```python
from build123d import *

# Parameters (mm, degrees)
F0_W        = 34.925
F0_H        = 25.4
F1_DEPTH    = 3.1496
F2_SIZE     = 3.14959
F3_W        = 29.1948509403
F3_H        = 13.3209023625
F4_DEPTH    = 25.4
F5_T        = 2.54
F5_T3_DEPTH = 34.2748509403
F5_T5_DEPTH = 18.4009023625


# Not quite as in the source:
# - a fillet or chamfer is up to 0.001 mm smaller than in the source, because OpenCascade refuses the exact size
# - a shell that OpenCascade refuses in one call is made with other operations: the cavity is built on its own and cut out


with BuildPart() as f1:
    # F0 (on Top) → F1 (new body)
    with BuildSketch(Plane.XY):
        with Locations((9.7498925388, -19.8326882303)):
            Rectangle(F0_W, F0_H)
    extrude(amount=F1_DEPTH)

    # F2 (size 3.1496 in the source; OpenCascade refuses exactly that, so slightly less here)
    f2_edges = [f1.edges().sort_by_distance(p)[0] for p in [
        (9.749893, -32.532688, 3.1496),
        (9.749893, -7.132688, 3.1496),
    ]]
    chamfer(f2_edges, length=F2_SIZE)

    # F3 (on face) → F4 (join)
    with BuildSketch(Plane.XY.offset(3.1496)):
        with Locations((8.8992563542, -19.3738183007)):
            Rectangle(F3_W, F3_H)
    extrude(amount=F4_DEPTH)

    # F5: shell of thickness 2.54, made by hand


with BuildPart() as f5_core1:
    # F5_t2: copy of F1
    add(f1.part)

    # the walls: a layer under each face that stays
    f5_faces = [f5_core1.faces().sort_by_distance(p)[0] for p in [
        (27.2123925388, -19.8326882303, 1.5748),
        (9.7498925388, -32.5326882303, 5e-06),
        (9.7498925388, -30.9578932303, 1.574805),
        (9.7498925388, -19.8326882303, 0),
        (-1.8917741279, -26.1996282303, 3.1496),
        (9.7498925388, -7.1326882303, 5e-06),
        (9.7498925388, -8.7074832303, 1.574805),
        (-7.7126074612, -19.8326882303, 1.5748),
        (8.8992563542, -12.7133671194, 15.8496),
        (-5.6981691159, -19.3738183007, 15.8496),
        (8.8992563542, -26.0342694819, 15.8496),
        (23.4966818243, -19.3738183007, 15.8496),
    ]]
    thicken(f5_faces, amount=-F5_T, mode=Mode.SUBTRACT)

    # F5_s4 → F5_t3 (cut)
    with BuildSketch(Plane.YZ.offset(-8.2381691159)):
        Polygon((-12.6879671194, 3.175), (-12.7133671194, 0.6096), (-15.2533671194, 0.6096), (-15.2533671194, 3.1496), align=None)
        Polygon((-26.0596694819, 3.175), (-26.0342694819, 0.6096), (-23.4942694819, 0.6096), (-23.4942694819, 3.1496), align=None)
    extrude(amount=F5_T3_DEPTH, mode=Mode.SUBTRACT)

    # F5_s6 → F5_t5 (cut)
    with BuildSketch(Plane.XZ.offset(10.1733671194)):
        Polygon((-5.7235691159, 3.175), (-5.6981691159, 0.6096), (-3.1581691159, 0.6096), (-3.1581691159, 3.1496), align=None)
        Polygon((23.5220818243, 3.175), (23.4966818243, 0.6096), (20.9566818243, 0.6096), (20.9566818243, 3.1496), align=None)
    extrude(amount=F5_T5_DEPTH, mode=Mode.SUBTRACT)


with BuildPart() as f1_1:
    add(f1.part)

    # what is left inside the walls is the cavity
    f5_cavity = [f5_core1.part.solids().sort_by_distance(p)[0] for p in [
        (12.918398, -15.278767, 15.5448),
    ]]
    add(f5_cavity, mode=Mode.SUBTRACT)


solid = f1_1.part
```
Part model, mm, in its own coordinate system. A direction names the side the tool comes from. Give positions to 0.01 mm unless a question says otherwise; leave off trailing zeros. Write each loop counter-clockwise with the first axis right and the second up, starting at its lowest first coordinate (ties: lowest second). Pieces come first, ordered by that corner, then holes. Notation, with made-up numbers: (-32.5, 68) -> (-23.5, 68) arc R24 ccw to (-23.5, 90) -> close; hole circle Ø2 at (-2.5, 53.25). An arc over 180 degrees is marked (long way). Put each result on its own line as item: value. Start each with the question number.
Item 1: Pull direction X, two halves, no side cores. Call faces 1 (the face through (-5.698, -19, 16)), 2 (the face through (9.51, -8.73, 1.6)), 3 (the face through (9, -15.253, 15)): pulls with the +X half, pulls with the -X half, needs draft (parallel to the pull), parting line crosses it, or undercut.
Item 2: Pin check, flat tips, straight feed: pin 1 Ø4 at (x, z) = (13, 21.5) entering from -Y; pin 2 Ø5 at (y, z) = (-17, 15) entering from +X; pin 3 Ø8 at (y, z) = (-21.5, 18) entering from -X. Stop position of each tip, or through.
Item 3: Wall check: L1, parallel to Y at x = 0.5, z = 26.25; L2, parallel to X at y = -17, z = 19; L3, parallel to Z at x = 20, y = -11.75. Give the ranges that are in metal, low to high. Write a range as [from, to].
Item 4: Which spindle directions (+Z, -Z, +X, -X, +Y, -Y) get a long thin tool onto all of the face, cutting with end or side? Do faces 4 (the face through (9, -23.494, 15)), 5 (the face through (23.497, -19, 16)), 6 (the face through (9, -26.034, 16)), 7 (the face through (9, -12.713, 16)). Say none if no direction does.
Item 5: Cut at C-C (y = -17). List the corners of the cut face in (x, z).
Item 6: Cut at A-A (z = 17.5). List the corners of the cut face in (x, y), then the cut area to 3 significant figures.
Answer list:
1. face 1: pulls with the -X half
1. face 2: needs draft
1. face 3: undercut
2. pin 1: stops at y = -26.03
2. pin 2: stops at x = 23.5
2. pin 3: stops at x = -5.7
3. L1: y = [-26.03, -23.49], [-15.25, -12.71]
3. L2: x = [-5.7, -3.16], [20.96, 23.5]
3. L3: z = [0, 3.15]
4. face 4: +Z
4. face 5: +Z, +X, +Y, -Y
4. face 6: +Z, +X, -X, -Y
4. face 7: +Z, +X, -X, +Y
5. outline: (-7.71, 0) -> (27.21, 0) -> (27.21, 3.15) -> (23.5, 3.15) -> (23.5, 28.55) -> (20.96, 28.55) -> (20.96, 2.54) -> (-3.16, 2.54) -> (-3.16, 28.55) -> (-5.7, 28.55) -> (-5.7, 3.15) -> (-7.71, 3.15) -> close
6. outline: (-5.7, -26.03) -> (23.5, -26.03) -> (23.5, -12.71) -> (-5.7, -12.71) -> close; hole (-3.16, -23.49) -> (20.96, -23.49) -> (20.96, -15.25) -> (-3.16, -15.25) -> close
6. area: 190 mm2
